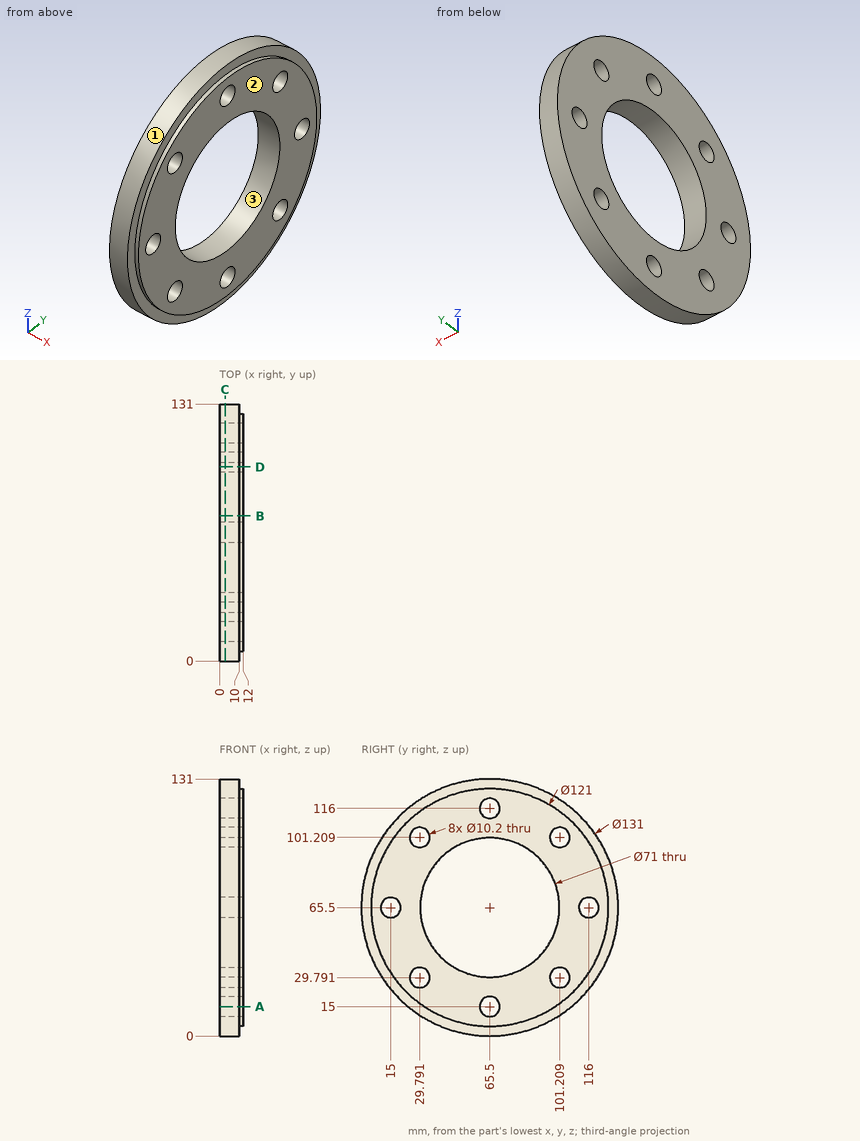
Check sheet for the drawn part. Datum: minimum x, y, z corner. Units: mm. Coordinates: 2 decimals unless noted, no trailing zeros. Loops run counter-clockwise (first coordinate to the right, second up) from the corner with the lowest first, then second, coordinate; pieces in that order, holes last. Notation, with made-up numbers: (42, 47) -> (62, 47) arc R7 ccw to (62, 53) -> close; hole circle Ø11 at (13.25, 11.5). An arc over 180 degrees is marked (long way). Answer as a JSON object with one key per item and string values. Group by question number.
Item 1: Mould release check, pull along Y, two halves, no side actions. Record for the marked faces 1, 2 and 3: +Y half, -Y half, draft (parallel to the pull), parting line (faces both ways), or undercut.
Item 2: Sectioned sample at A-A on z = 15. Record the boundary of the cut face in (x, y), plus the area to 3 significant figures.
Item 3: Scan lines: probe 1 along Y at (x, z) = (8.25, 65.5); probe 2 along Y at (x, z) = (3.5, 98) (1 decimal); probe 3 along X at (y, z) = (41, 121). Record each from-to range of solid material in increasing order.
Item 4: Sectioned sample at B-B on y = 74. Record the boundary of the cut face in (x, z), plus the area to 3 significant figures.
Item 5: Depth check by flat-ended pin: pin 1 (2 mm diameter, centred on x = 3.5, y = 114, fed in from -Z); pin 2 (11.5 mm diameter, centred on y = 101.21, z = 101.21, fed in from -X); pin 3 (4 mm diameter, centred on x = 6.5, y = 42.5, fed in from -Z); pin 4 (1.5 mm diameter, centred on x = 10.5, y = 97, fed in from -Z). Enter the tip coordinate at first touch or a pass-through.
Item 6: Sectioned sample at C-C on x = 2.75. State how many separate pieces and enclosed holes the cut face has, plus the area to 3 significant figures.
Item 7: Sectioned sample at D-D on y = 99. Record the boundary of the cut face in (x, z) (1 decimal), plus the area to 3 significant figures.
Evaluation:
{
 "1": {"face 1": "parting line", "face 2": "draft", "face 3": "undercut"},
 "2": {"outline": "(0, 23.79) -> (10, 23.79) -> (10, 32.18) -> (12, 32.18) -> (12, 60.4) -> (0, 60.4) -> close; (0, 70.6) -> (12, 70.6) -> (12, 98.82) -> (10, 98.82) -> (10, 107.21) -> (0, 107.21) -> close", "area": "845 mm²"},
 "3": {"probe 1": "y = 0 to 9.9, 20.1 to 30, 101 to 110.9, 121.1 to 131", "probe 2": "y = 8.6 to 25.8, 33.8 to 51.2, 79.8 to 97.2, 105.2 to 122.4", "probe 3": "x = 0 to 10"},
 "4": {"outline": "(0, 0.55) -> (10, 0.55) -> (10, 5.6) -> (12, 5.6) -> (12, 31.03) -> (0, 31.03) -> close; (0, 99.97) -> (12, 99.97) -> (12, 125.4) -> (10, 125.4) -> (10, 130.45) -> (0, 130.45) -> close", "area": "711 mm²"},
 "5": {"pin 1": "stops at z = 20.4", "pin 2": "stops at x = 0", "pin 3": "stops at z = 3.46", "pin 4": "stops at z = 7.77"},
 "6": {"separate pieces": "1", "enclosed holes": "9", "area": "8,870 mm²"},
 "7": {"outline": "(0, 9.2) -> (10, 9.2) -> (10, 15.1) -> (12, 15.1) -> (12, 25.2) -> (0, 25.2) -> close; (0, 34.4) -> (12, 34.4) -> (12, 53.8) -> (0, 53.8) -> close; (0, 77.2) -> (12, 77.2) -> (12, 96.6) -> (0, 96.6) -> close; (0, 105.8) -> (12, 105.8) -> (12, 115.9) -> (10, 115.9) -> (10, 121.8) -> (0, 121.8) -> close", "area": "825 mm²"}
}
